from build123d import *

# Parameters (mm, degrees)
SKETCH1_W                               = 55.000000074
SKETCH1_H                               = 16.2630756
BOSS_EXTRUDE1_DEPTH                     = 5
SKETCH4_W                               = 15
SKETCH4_H                               = 14
BOSS_EXTRUDE2_DEPTH                     = 5
CBORE_FOR_M6_HEX_HEAD_BOLT1_D           = 6.647
CBORE_FOR_M6_HEX_HEAD_BOLT1_DEPTH       = 10
CBORE_FOR_M6_HEX_HEAD_BOLT1_CBORE_D     = 9
CBORE_FOR_M6_HEX_HEAD_BOLT1_CBORE_DEPTH = 2
CBORE_FOR_M6_HEX_HEAD_BOLT1_TIP         = 1.996960267
FILLET1_R                               = 1
FILLET2_R                               = 4
TAP_DRILL_FOR_M3X0_5_TAP1_D             = 2.5


with BuildPart() as part:
    # Sketch1 → Boss-Extrude1 (new body)
    with BuildSketch(Plane(origin=(0, 0, 0), x_dir=(-1, 0, 0), z_dir=(0, 0, -1))):
        with Locations((3.7e-08, -8.131537807)):
            Rectangle(SKETCH1_W, SKETCH1_H)
    extrude(amount=-BOSS_EXTRUDE1_DEPTH)

    # Sketch4 → Boss-Extrude2 (add)
    with BuildSketch(Plane.XY.offset(5)):
        with Locations((0, -7)):
            Rectangle(SKETCH4_W, SKETCH4_H)
    extrude(amount=BOSS_EXTRUDE2_DEPTH)

    # CBORE for M6 Hex Head Bolt1
    with Locations(Plane(origin=(0, 0, 0), x_dir=(1, 0, 0), z_dir=(0, 1, 0))):
        with Locations((0, -5)):
            CounterBoreHole(CBORE_FOR_M6_HEX_HEAD_BOLT1_D / 2, CBORE_FOR_M6_HEX_HEAD_BOLT1_CBORE_D / 2, CBORE_FOR_M6_HEX_HEAD_BOLT1_CBORE_DEPTH, depth=CBORE_FOR_M6_HEX_HEAD_BOLT1_DEPTH)
            with Locations((0, 0, -(CBORE_FOR_M6_HEX_HEAD_BOLT1_DEPTH + CBORE_FOR_M6_HEX_HEAD_BOLT1_TIP / 2))):  # 118° drill point
                Cone(0, CBORE_FOR_M6_HEX_HEAD_BOLT1_D / 2, CBORE_FOR_M6_HEX_HEAD_BOLT1_TIP, mode=Mode.SUBTRACT)

    # Fillet1
    fillet1_edges = [part.edges().sort_by_distance(p)[0] for p in [
        (27.5, -7e-09, 2.5),
        (-27.500000074, -7e-09, 2.5),
        (27.5, -16.263075607, 2.5),
        (-27.500000074, -16.263075607, 2.5),
    ]]
    fillet(fillet1_edges, radius=FILLET1_R)

    # Fillet2
    fillet2_edges = [part.edges().sort_by_distance(p)[0] for p in [
        (7.5, -14, 7.5),
        (7.5, -7, 10),
        (-7.5, -14, 7.5),
        (0, -14, 10),
        (-7.5, -7, 10),
    ]]
    fillet(fillet2_edges, radius=FILLET2_R)

    # Tap Drill for M3x0.5 Tap1 (through all)
    with Locations(Plane(origin=(-10.5, -2.500000007, 5), x_dir=(1, 0, 0), z_dir=(0, 0, 1))):
        with Locations((0, 0), (21, 0)):
            Hole(TAP_DRILL_FOR_M3X0_5_TAP1_D / 2)


solid = part.part
Could you check a few things on this model? Use its own coordinates, in mm. A direction names the side the tool comes from. Round coordinates to 2 decimals unless told otherwise and drop trailing zeros. Loops run counter-clockwise (first coordinate to the right, second up) from the corner with the lowest first, then second, coordinate; pieces in that order, holes last. Notation, with made-up numbers: (-16.5, 68.5) - (25.5, 68.5) arc R29 ccw to (25.5, 94.5) - close; hole circle Ø10 at (-4, 30). An arc over 180 degrees is marked (long way). Write item = value, one per line.
1) Imagine slicing it at C-C (x = -10.5). Please give me the cut outline in (y, z), and give its area (3 significant figures).
Computed:
outline = (-16.26, 0) - (-3.75, 0) - (-3.75, 5) - (-16.26, 5) - close; (-1.25, 0) - (0, 0) - (0, 5) - (-1.25, 5) - close
area = 68.8 mm2
2) If we mould it in two halves opening along Z, with no side actions, what happens to faces 4 (the conical face through (-0.08, -11.65, 4.43)), 5 (the flat face through (0, -14, 5.5)), 6 (the flat face through (0, -8, 0))? For each: pulls with the +Z half, pulls with the -Z half, needs draft (parallel to the pull), parting line crosses it, or undercut.
Computed:
face_4 = undercut
face_5 = needs draft
face_6 = pulls with the -Z half
3) Imagine slicing it at B-B (y = -6). Please give me the cut outline in (x, z), and give its area (3 significant figures).
Computed:
outline = (-27.5, 0) - (27.5, 0) - (27.5, 5) - (7.5, 5) - (7.5, 6) arc R4 ccw to (3.5, 10) - (-3.5, 10) arc R4 ccw to (-7.5, 6) - (-7.5, 5) - (-27.5, 5) - close; hole circle Ø6.65 at (0, 5)
area = 308 mm2
4) On a 3-axis mill with a long thin cutter (end or side, diameter ignored), from which of +Z, -Z, +X, -X, +Y, -Y can I reach the whole of each face in a straight line? I mean faces 1 (the cylindrical face through (6.359, -12.797, 5.507)), 2 (the cylindrical face through (-6.297, -12.859, 5.507)), 3 (the flat face through (-7.5, -5.1, 5.5)). Say none if no direction works.
Computed:
face_1 = +Z, +X, -Y
face_2 = +Z, -X, -Y
face_3 = +Z, -X, +Y, -Y
5) Imagine slicing it at D-D (z = 9). Please give me the cut outline in (x, y), and give its area (3 significant figures).
Computed:
outline = (-6.15, -10) arc R2.65 ccw to (-3.5, -12.65) - (3.5, -12.65) arc R2.65 ccw to (6.15, -10) - (6.15, 0) - (2.06, 0) - (2.06, -2) - (-2.06, -2) - (-2.06, 0) - (-6.15, 0) - close
area = 144 mm2
6) I'm going to push flat-ended pins straight in: P1, Ø1, axis at y = -3, z = 9, coming from the +X side; P2, Ø3, axis at x = -10.5, y = -2.5, coming from the +Z side; P3, Ø0.5, axis at y = -3.5, z = 5.5, coming from the +X side. Where does each tip first touch, or does it pass through?
Computed:
P1 = 6.62
P2 = 5
P3 = 7.5
7) I need wall thicknesses on line 1 along X through (y, z) = (-3.75, 5.25); line 2 along Y through (x, z) = (10.5, 2.35); line 3 along Z through (x, y) = (0, -5). Which ranges of each line are inside material? Lowest first, please. Write a range as from..to.
Computed:
line_1 = -7.5..-3.31, 3.31..7.5
line_2 = -16.26..-3.75, -1.25..0
line_3 = 0..1.68, 8.32..10
8) Imagine slicing it at A-A (y = -2.5). Please give me the cut outline in (x, z).
Computed:
outline = (-27.5, 0) - (-11.75, 0) - (-11.75, 5) - (-27.5, 5) - close; (-9.25, 0) - (9.25, 0) - (9.25, 5) - (7.5, 5) - (7.5, 6) arc R4 ccw to (3.5, 10) - (-3.5, 10) arc R4 ccw to (-7.5, 6) - (-7.5, 5) - (-9.25, 5) - close; (11.75, 0) - (27.5, 0) - (27.5, 5) - (11.75, 5) - close; hole circle Ø6.65 at (0, 5)
